Read the model definition and answer for the solid it produces. Units are mm, in the model's axes. A direction names the side the tool comes from. Coordinates: 2 decimals unless noted, no trailing zeros. Write each loop counter-clockwise with the first axis right and the second up, starting at its lowest first coordinate (ties: lowest second). Pieces come first, ordered by that corner, then holes. Notation, with made-up numbers: (-31.5, 21.25) -> (27.5, 21.25) arc R20 cw to (27.5, 34.25) -> close; hole circle Ø8 at (51, -20.75). An arc over 180 degrees is marked (long way). Use CSV: the item, a comma, the result in double quotes. Start each with the question number.
from build123d import *

# Parameters (mm, degrees)
SKETCH1_R           = 16
BOSS_EXTRUDE1_DEPTH = 67.12
BOSS_EXTRUDE2_START = -67.12
SKETCH2_R           = 17
SKETCH2_R_2         = 16
BOSS_EXTRUDE2_DEPTH = 5
FILLET1_R           = 0.5


with BuildPart() as part:
    # Sketch1 → Boss-Extrude1 (new body)
    with BuildSketch(Plane(origin=(0, 0, 0), x_dir=(1, 0, 0), z_dir=(0, 1, 0))):
        Circle(SKETCH1_R)
    extrude(amount=BOSS_EXTRUDE1_DEPTH)

    # Sketch2 → Boss-Extrude2 (add)
    with BuildSketch(Plane.XZ.offset(BOSS_EXTRUDE2_START)):
        Circle(SKETCH2_R)
        Circle(SKETCH2_R_2, mode=Mode.SUBTRACT)
    extrude(amount=BOSS_EXTRUDE2_DEPTH)

    # Fillet1
    fillet1_edges = [part.edges().sort_by_distance(p)[0] for p in [
        (-16, 0, 0),
        (-17, 62.12, 0),
        (-17, 67.12, 0),
    ]]
    fillet(fillet1_edges, radius=FILLET1_R)


solid = part.part
1) Each of these flat-tipped pins is pushed along its axis until it touches: pin 1 (10 mm diameter, centred on y = 33, z = -12, fed in from +X); pin 2 (5 mm diameter, centred on x = 10.5, y = 31.5, fed in from -Z); pin 3 (2 mm diameter, centred on x = -12, y = 48, fed in from +Z); pin 4 (10 mm diameter, centred on x = 11.5, z = -12, fed in from +Y). Where does it stop, or does it pass through?
2) Find the intervals of material crossed by line 1 along X through (y, z) = (3.5, -0.5); line 2 along X through (y, z) = (48.5, -1.5); line 3 along Z through (x, y) = (12.5, 30.5), in increasing order.
3) Section A-A, the plane x = 0 is taken. Give the vertices of the cut face in (y, z).
4) Section C-C, the plane y = 52 is taken. Give the vertices of the cut face in (x, z), plus the area to 3 significant figures.
5) Section B-B, the plane z = 0 is taken. Give the vertices of the cut face in (x, y).
6) Which of the six approach directions +Z, -Z, +X, -X, +Y, -Y give full straight-line access (tool end or side, diameter ignored) to faces 1 (the face through (0, 67.12, 0)), 2 (the face through (-16, 62.12, 3))?
The answers:
1,pin 1,"stops at x = 14.39"
1,pin 2,"stops at z = -13.86"
1,pin 3,"stops at z = 11.62"
1,pin 4,"stops at y = 67.12"
2,line 1,"x = -15.99 to 15.99"
2,line 2,"x = -15.93 to 15.93"
2,line 3,"z = -9.99 to 9.99"
3,outline,"(0, -15.5) arc R0.5 ccw to (0.5, -16) -> (62.12, -16) -> (62.12, -16.5) arc R0.5 ccw to (62.62, -17) -> (66.62, -17) arc R0.5 ccw to (67.12, -16.5) -> (67.12, 16.5) arc R0.5 ccw to (66.62, 17) -> (62.62, 17) arc R0.5 ccw to (62.12, 16.5) -> (62.12, 16) -> (0.5, 16) arc R0.5 ccw to (0, 15.5) -> close"
4,outline,"circle Ø32 at (0, 0)"
4,area,"804 mm^2"
5,outline,"(-17, 62.62) arc R0.5 ccw to (-16.5, 62.12) -> (-16, 62.12) -> (-16, 0.5) arc R0.5 ccw to (-15.5, 0) -> (15.5, 0) arc R0.5 ccw to (16, 0.5) -> (16, 62.12) -> (16.5, 62.12) arc R0.5 ccw to (17, 62.62) -> (17, 66.62) arc R0.5 ccw to (16.5, 67.12) -> (-16.5, 67.12) arc R0.5 ccw to (-17, 66.62) -> close"
6,face 1,"+Z, -Z, +X, -X, +Y"
6,face 2,"-Y"
